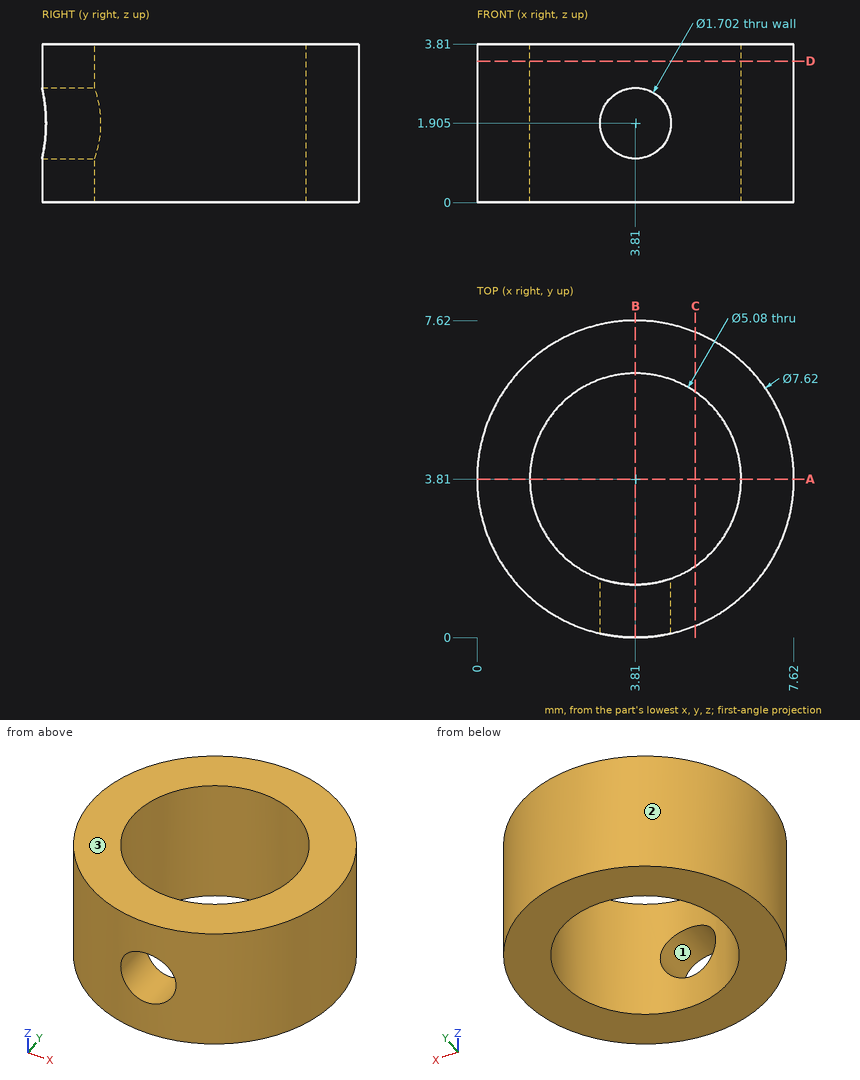
The drawing under review shows one solid part. Ordinate dimensions are in mm from its lowest x, y, z. Round coordinates to 2 decimals unless told otherwise and drop trailing zeros. Write each loop counter-clockwise with the first axis right and the second up, starting at its lowest first coordinate (ties: lowest second). Pieces come first, ordered by that corner, then holes. Notation, with made-up numbers: M 34,14.5 L 70,14.5 A24 cw 70,24.5 Z; hole C 42,39 d7. An arc over 180 degrees is marked long. One line per item, written item: value. Start each with the question number.
(1) Insertion check: pin 1 (1 mm diameter, centred on x = 1, z = 1.5, fed in from -Y); pin 2 (1.5 mm diameter, centred on x = 1, z = 3.5, fed in from +Y) (1 decimal). Each pin has a flat end and moves straight along its axis. Give the tip position at first contact, or say it passes through.
(2) We need section D-D (z = 3.4). Give the boundary of the cut face in (x, y).
(3) The part is to be moulded in two halves that separate along X. For the marked faces 1, 2 and 3, say which applies: released by +X, released by -X, zero draft, split by the parting line, or undercut.
(4) We need section C-C (x = 5.25). Give the boundary of the cut face in (y, z).
(5) We need section A-A (y = 3.81). Give the boundary of the cut face in (x, z).
(6) Wall thickness on line 1 (X direction, y = 3.5, z = 2.2); line 2 (Y direction, x = 5.5, z = 0.85) (1 decimal); line 3 (Y direction, x = 6, z = 3.05) (1 decimal): over which ranges is each line inside the solid? List them lowest first.
(7) We need section B-B (x = 3.81). Give the boundary of the cut face in (y, z).
Result:
1. pin 1: y = 0.78
1. pin 2: y = 7
2. outline: C 3.81,3.81 d7.62; hole C 3.81,3.81 d5.08
3. face 1: undercut
3. face 2: split by the parting line
3. face 3: zero draft
4. outline: M 0.28,0 L 1.72,0 L 1.72,3.81 L 0.28,3.81 Z; M 5.9,0 L 7.34,0 L 7.34,3.81 L 5.9,3.81 Z
5. outline: M 0,0 L 1.27,0 L 1.27,3.81 L 0,3.81 Z; M 6.35,0 L 7.62,0 L 7.62,3.81 L 6.35,3.81 Z
6. line 1: 0.01 to 1.29, 6.33 to 7.61
6. line 2: 0.4 to 1.9, 5.7 to 7.2
6. line 3: 0.7 to 2.5, 5.1 to 6.9
7. outline: M 0,0 L 1.27,0 L 1.27,1.05 L 0,1.05 Z; M 0,2.76 L 1.27,2.76 L 1.27,3.81 L 0,3.81 Z; M 6.35,0 L 7.62,0 L 7.62,3.81 L 6.35,3.81 Z
